Part model, mm, in its own coordinate system. Face numbers are marked on the shaded views. A direction names the side the tool comes from. Give positions to 0.01 mm unless a question says otherwise; leave off trailing zeros. Write each loop counter-clockwise with the first axis right and the second up, starting at its lowest first coordinate (ties: lowest second). Pieces come first, ordered by that corner, then holes. Notation, with made-up numbers: M -40,65 L 17,65 A15 ccw 17,70 Z; hole C 26,72 d7. An arc over 180 degrees is marked long. Answer as CSV lines item,"result". Start each with the question number.
1) Tool access for the marked faces 5, 6 and 7: list every direction of +Z, -Z, +X, -X, +Y, -Y with a clear straight run to the whole face (end or side of a thin tool).
2) Pin check, flat tips, straight feed: pin 1 Ø1.5 at (x, y) = (-11.5, -38) entering from +Z; pin 2 Ø4.5 at (y, z) = (-53.5, 37) entering from +X; pin 3 Ø4 at (y, z) = (-3, 33.5) entering from +X. Stop position of each tip, or through.
3) Mould opens along X. For the marked faces 1, 2, 3 and 4 say: pulls with the +X half, pulls with the -X half, needs draft (parallel to the pull), parting line crosses it, or undercut.
4) Slice it at D-D, the plane y = -35. Give the cut face in (x, z), plus the area to 4 significant figures.
5) Slice it at B-B, the plane y = 10. Give the cut face in (x, z), plus the area to 3 significant figures.
6) Wall check: line 1 along X through (y, z) = (10, 29.5); line 2 along Z through (x, y) = (-36, -2); line 3 along Y through (x, z) = (-9, 42). Give the ranges that are in metal, low to high. Write a range as from..to.
7) Slice it at A-A, the plane x = -40. Give the cut face in (y, z).
8) Slice it at C-C, the plane z = 33.5. Give the cut face in (x, y), plus the area to 3 significant figures.
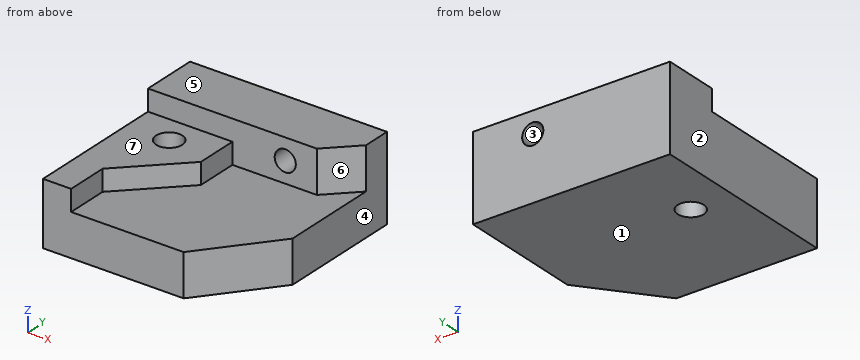
Autodesk Fusion 360 part; units mm, degrees
sketch "Sketch1" plane through (0, 0, 0) normal (0, 0, 1) x (1, 0, 0) in component "box"
  line L0 (70, 70) -> (-70, 70)
  line L1 (-70, 70) -> (-70, -70)
  line L2 (-70, -70) -> (70, -70)
  line L3 (70, -70) -> (70, 70)
  line L4 (70, 70) -> (-70, -70) construction
  line L5 (-70, 70) -> (70, -70) construction
  dimension "d1" = 140
extrude "Extrude1" add sketch "Sketch1" along normal blind 30 in component "box"
sketch "Sketch2" plane through (0, -70, 0) normal (0, -1, 0) x (1, 0, 0) in component "box"
  line L0 (-70, 0) -> (70, 0)
  line L1 (70, 0) -> (70, 30)
  line L2 (70, 30) -> (-70, 30)
  line L3 (-70, 30) -> (-70, 0)
sketch "Sketch3" plane through (0, 0, 30) normal (0, 0, 1) x (-1, 0, 0) in component "box"
  line L0 (-70, 70) -> (-70, -70)
  line L1 (-70, -70) -> (70, -70)
  line L2 (70, -70) -> (70, 70)
  line L3 (70, 70) -> (-70, 70)
  line L4 (-70, 20) -> (-30, 70)
  line L5 (-30, 70) -> (-70, 70)
  line L6 (-70, 20) -> (-70, 70)
extrude "Extrude2" cut sketch "Sketch3" against normal up to surface (30 mm away) contours L0 L3 L4 L5 L6 in component "box"
sketch "Sketch4" plane through (0, 0, 30) normal (0, 0, 1) x (-1, 0, 0) in component "box"
  line L0 (-30, 70) -> (-70, 20)
  line L1 (-70, 20) -> (-70, -70)
  line L2 (-70, -70) -> (70, -70)
  line L3 (70, -70) -> (70, 70)
  line L4 (70, 70) -> (-30, 70)
  line L5 (-70, -30) -> (70, -30)
  line L6 (70, -30) -> (70, -70)
  line L7 (70, -70) -> (-70, -70)
  line L8 (-70, -70) -> (-70, -30)
  line L9 (-70, -30) -> (70, -70) construction
  line L10 (70, -30) -> (-70, -70) construction
  point P0 (0, -50)
extrude "Extrude3" add sketch "Sketch4" along normal blind 30 contours L1 L2 L3 L5 L6 L7 L8 in component "box"
sketch "Sketch5" plane through (0, 0, 30) normal (0, 0, 1) x (-1, 0, 0) in component "box"
  line L0 (-70, -30) -> (70, -30)
  line L1 (70, -30) -> (70, 70)
  line L2 (70, 70) -> (-30, 70)
  line L3 (-30, 70) -> (-70, 20)
  line L4 (-70, 20) -> (-70, -30)
  line L5 (10, -30) -> (70, -30)
  line L6 (70, -30) -> (70, 70)
  line L7 (70, 70) -> (10, 70)
  line L8 (10, 70) -> (10, -30)
  line L9 (10, -30) -> (70, 70) construction
  line L10 (70, -30) -> (10, 70) construction
  point P0 (40, 20)
extrude "Extrude4" add sketch "Sketch5" along normal blind 15 contours L0 L1 L2 L5 L6 L7 L8 in component "box"
sketch "Sketch6" plane through (0, 0, 45) normal (0, 0, 1) x (-1, 0, 0) in component "box"
  line L0 (10, 70) -> (10, -30)
  line L1 (10, -30) -> (70, -30)
  line L2 (70, -30) -> (70, 70)
  line L3 (70, 70) -> (10, 70)
  line L4 (50, 70) -> (50, 40)
  line L5 (50, 40) -> (10, 0)
  line L6 (10, 70) -> (50, 70)
extrude "Extrude5" cut sketch "Sketch6" against normal blind 15 contours L0 L3 L4 L5 L6 in component "box"
sketch "Sketch7" plane through (0, 0, 60) normal (0, 0, 1) x (-1, 0, 0) in component "box"
  line L0 (-70, -70) -> (70, -70)
  line L1 (70, -70) -> (70, -30)
  line L2 (70, -30) -> (-70, -30)
  line L3 (-70, -30) -> (-70, -70)
  line L4 (-70, -50) -> (-50, -30)
  line L5 (-70, -30) -> (-70, -50)
extrude "Extrude6" cut sketch "Sketch7" against normal blind 30 contours L2 L3 L4 L5 in component "box"
sketch "Sketch8" plane through (0, 0, 45) normal (0, 0, 1) x (-1, 0, 0) in component "box"
  line L0 (50, 40) -> (10, 0)
  line L1 (10, 0) -> (10, -30)
  line L2 (10, -30) -> (70, -30)
  line L3 (70, -30) -> (70, 70)
  line L4 (70, 70) -> (50, 70)
  line L5 (50, 70) -> (50, 40)
  circle A0 centre (40, -10) radius 9.3121
extrude "Extrude7" cut sketch "Sketch8" against normal blind 45 contours A0 in component "box"
sketch "Sketch9" plane through (0, 30, 0) normal (0, -1, 0) x (1, 0, 0) in component "box"
  line L0 (50, 30) -> (50, 60)
  line L1 (50, 60) -> (-70, 60)
  line L2 (-70, 60) -> (-70, 45)
  line L3 (-70, 45) -> (-10, 45)
  line L4 (-10, 45) -> (-10, 30)
  line L5 (-10, 30) -> (50, 30)
  circle A0 centre (27.54, 44.8379) radius 7.5144
extrude "Extrude8" cut sketch "Sketch9" against normal blind 40 contours A0 in component "box"
component "box" placed x (1, 0, 0) y (0, 1, 0) z (0, 0, 1) at (0, 0, 0)
Found:
1,face 5,"+Z, +X, -X, +Y, -Y"
1,face 6,"+Z, +X, -Y"
1,face 7,"+Z, +X, -X, -Y"
2,pin 1,"z = 30"
2,pin 2,"x = -50"
2,pin 3,"x = -11"
3,face 1,"needs draft"
3,face 2,"pulls with the -X half"
3,face 3,"undercut"
3,face 4,"pulls with the +X half"
4,outline,"M -70,0 L 58,0 L 58,30 L -45,30 L -45,45 L -70,45 Z"
4,area,"4,215 mm²"
5,outline,"M -70,0 L -49.31,0 L -49.31,45 L -70,45 Z; M -30.69,0 L 70,0 L 70,30 L -10,30 L -10,45 L -30.69,45 Z"
5,area,"4,260 mm²"
6,line 1,"-70..-49.31, -30.69..70"
6,line 2,"0..45"
6,line 3,"30..70"
7,outline,"M -70,0 L 0.69,0 L 0.69,45 L -30,45 L -30,30 L -70,30 Z; M 19.31,0 L 70,0 L 70,60 L 30,60 L 30,45 L 19.31,45 Z"
8,outline,"M -70,-70 L -50,-70 L -50,-40 L -10,0 L -10,30 L 50,30 L 70,50 L 70,70 L -70,70 Z; hole C -40,10 d18.62"
8,area,"9,130 mm²"
